Autodesk Inventor part; units mm, degrees
ref_plane "YZ Plane" through (0, 0, 0) normal (1, 0, 0) x (0, 1, 0)
ref_plane "XZ Plane" through (0, 0, 0) normal (0, 1, 0) x (-1, 0, 0)
ref_plane "XY Plane" through (0, 0, 0) normal (0, 0, 1) x (1, 0, 0)
sketch "Эскиз1" plane through (0, 0, 0) normal (0, 1, 0) x (-1, 0, 0)
  line L0 (-4, 17.5) -> (4, 17.5)
  line L1 (4, 3.5) -> (4, -17.5)
  line L2 (4, -17.5) -> (-4, -17.5)
  line L3 (-4, -17.5) -> (-4, 17.5)
  line L4 (-4, 17.5) -> (4, -17.5) construction
  line L5 (4, 17.5) -> (-4, -17.5) construction
  line L6 (4, 17.5) -> (19, 17.5)
  line L7 (19, 17.5) -> (19, 9.5)
  line L8 (19, 9.5) -> (10, 9.5)
  arc A0 (10, 9.5) -> (4, 3.5) centre (10, 3.5) ccw
  point P0 (0, 0)
  point P1 (4, 9.5)
  dimension "d0" = 8
  dimension "d2" = 15
  dimension "d3" = 8
  dimension "d4" = 35
  dimension "d5" = 6
extrude "Выдавливание1" add sketch "Эскиз1" along normal blind 9
properties part number "angle"
Model file for the job. Use its own axes, mm. A direction names the side the tool comes from. Coordinates: 2 decimals unless noted, no trailing zeros. Write each loop counter-clockwise with the first axis right and the second up, starting at its lowest first coordinate (ties: lowest second). Pieces come first, ordered by that corner, then holes. Notation, with made-up numbers: (-13.75, -2.75) - (5.25, -2.75) arc R21 cw to (5.25, 24.25) - close; hole circle Ø8 at (71, 5). An arc over 180 degrees is marked (long way). One line per question, with ' | ' between items. Start each with the question number.
Q1. Cut at A-A, the plane y = 1. List the corners of the cut face in (x, z).
Q2. Cut at C-C, the plane z = -9.5. List the corners of the cut face in (x, y), then the cut area to 3 significant figures.
Q3. Cut at B-B, the plane x = -16.5. List the corners of the cut face in (y, z).
Q4. 3-axis set-ups, long thin cutter, end or side, ignore diameter. For faces 1 (the face through (-2, 0, 4)), 2 (the face through (-15, 4, 9.5)): which of +Z, -Z, +X, -X, +Y, -Y reach the whole face in a straight line?
Q5. Drill centre lines: line 1 (X direction, y = 2.75, z = -8); line 2 (Z direction, x = -10.25, y = 5); line 3 (Z direction, x = -7.5, y = 7.5). Where is each one in solid material? Low to high. Write a range as [from, to].
Q6. Pin check, flat tips, straight feed: pin 1 (2.5 mm diameter, centred on x = -14.5, y = 4.5, fed in from -Z); pin 2 (3 mm diameter, centred on y = 5, z = 1.5, fed in from -X). Stop position of each tip, or through.
Answer below:
1) outline: (-19, 9.5) - (-10, 9.5) arc R6 cw to (-4, 3.5) - (-4, -17.5) - (4, -17.5) - (4, 17.5) - (-19, 17.5) - close
2) outline: (-4, 0) - (4, 0) - (4, 9) - (-4, 9) - close | area: 72.0 mm^2
3) outline: (0, 9.5) - (9, 9.5) - (9, 17.5) - (0, 17.5) - close
4) face 1: +Z, -Z, +X, -X, -Y | face 2: -Z, -X, +Y, -Y
5) line 1: [-4, 4] | line 2: [9.5, 17.5] | line 3: [8.95, 17.5]
6) pin 1: z = 9.5 | pin 2: x = -4
